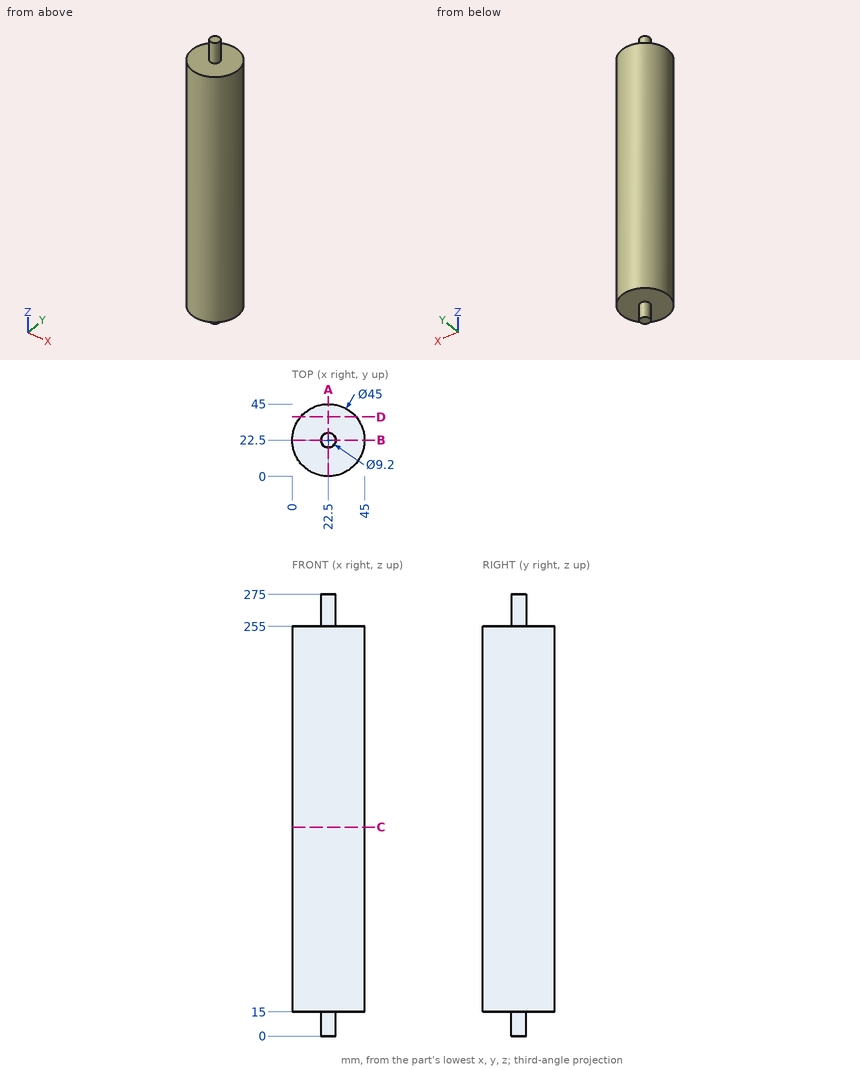
Geometry check sheet. Reference: drawing and pictorial views, mm from the part's lowest x, y, z. Round coordinates to 2 decimals unless told otherwise and drop trailing zeros. Loops run counter-clockwise (first coordinate to the right, second up) from the corner with the lowest first, then second, coordinate; pieces in that order, holes last.
1. Gauge pin test, flat ends, axial feed: pin 1 Ø6 at (y, z) = (36.5, 137) entering from -X; pin 2 Ø4 at (x, y) = (4.5, 7.5) entering from +Z; pin 3 Ø3 at (y, z) = (9, 127) entering from +X. Record the tip position at first contact, or that the pin passes through.
2. Sectioned sample at D-D on y = 37. Record the boundary of the cut face in (x, z).
3. Sectioned sample at A-A on x = 22.5. Record the boundary of the cut face in (y, z).
4. Sectioned sample at C-C on z = 130. Record the boundary of the cut face in (x, y), and give its area (3 significant figures).
5. Scan lines: probe 1 along Z at (x, y) = (5.5, 16.5); probe 2 along X at (y, z) = (24, 198); probe 3 along X at (y, z) = (22, 221.5). Record each from-to range of solid material in increasing order.
Recorded:
1. pin 1: stops at x = 2.87
1. pin 2: stops at z = 255
1. pin 3: stops at x = 41.53
2. outline: (5.3, 15) - (39.7, 15) - (39.7, 255) - (5.3, 255) - close
3. outline: (0, 15) - (17.9, 15) - (17.9, 0) - (27.1, 0) - (27.1, 15) - (45, 15) - (45, 255) - (27.1, 255) - (27.1, 275) - (17.9, 275) - (17.9, 255) - (0, 255) - close
4. outline: circle Ø45 at (22.5, 22.5)
4. area: 1,590 mm2
5. probe 1: z = 15 to 255
5. probe 2: x = 0.05 to 44.95
5. probe 3: x = 0.01 to 44.99
